Geometry check sheet. Reference: the model listing, model coordinates, mm. A direction names the side the tool comes from. Give positions to 0.01 mm unless a question says otherwise; leave off trailing zeros. Loops run counter-clockwise (first coordinate to the right, second up) from the corner with the lowest first, then second, coordinate; pieces in that order, holes last. Notation, with made-up numbers: (42.5, 51) -> (58.5, 51) arc R23 ccw to (58.5, 61) -> close; hole circle Ø1 at (36.5, 32.25). An arc over 180 degrees is marked (long way). Answer as a JSON object with one key per item and string values.
from build123d import *

# Parameters (mm, degrees)
BOSS_EXTRUDE1_DEPTH = 15
SKETCH2_R           = 10
BOSS_EXTRUDE2_DEPTH = 134
SKETCH4_R           = 7.25
CUT_EXTRUDE1_DEPTH  = 57
CUT_EXTRUDE2_DEPTH  = 93
SKETCH7_R           = 6.5
CUT_EXTRUDE3_DEPTH  = 6.6
SKETCH8_R           = 3.2
CUT_EXTRUDE4_DEPTH  = 9.4
FILLET1_R           = 0.25
CHAMFER1_SIZE       = 1
FILLET2_R           = 0.5
FILLET3_R           = 0.5
FILLET4_R           = 0.5
SKETCH9_R           = 3
CUT_EXTRUDE5_DEPTH  = 16
FILLET5_R           = 1


with BuildPart() as part:
    # Sketch1 → Boss-Extrude1 (new body)
    with BuildSketch(Plane(origin=(0, 0, 0), x_dir=(1, 0, 0), z_dir=(0, 1, 0))):
        with BuildLine():
            Line((17, -24.718414189), (17, 24.718414189))
            ThreePointArc((17, 24.718414189), (-30, 0), (17, -24.718414189))
        make_face()
    extrude(amount=BOSS_EXTRUDE1_DEPTH)

    # Sketch2 → Boss-Extrude2 (add)
    with BuildSketch(Plane(origin=(0, 15, 0), x_dir=(1, 0, 0), z_dir=(0, 1, 0))):
        Circle(SKETCH2_R)
    extrude(amount=BOSS_EXTRUDE2_DEPTH)

    # Sketch4 → Cut-Extrude1 (cut)
    with BuildSketch(Plane.XZ):
        Circle(SKETCH4_R)
    extrude(amount=-CUT_EXTRUDE1_DEPTH, mode=Mode.SUBTRACT)

    # Sketch5 → Cut-Extrude2 (cut, through all)
    with BuildSketch(Plane.XZ.offset(-57)):
        with BuildLine():
            Line((-4, 3), (4, 3))
            ThreePointArc((4, 3), (0, -5), (-4, 3))
        make_face()
    extrude(amount=-CUT_EXTRUDE2_DEPTH, mode=Mode.SUBTRACT)

    # Sketch7 → Cut-Extrude3 (cut)
    with BuildSketch(Plane(origin=(0, 15, 0), x_dir=(1, 0, 0), z_dir=(0, 1, 0))):
        with Locations((0, -20)):
            Circle(SKETCH7_R)
        with Locations((-20, 0)):
            Circle(SKETCH7_R)
        with Locations((0, 20)):
            Circle(SKETCH7_R)
    extrude(amount=-CUT_EXTRUDE3_DEPTH, mode=Mode.SUBTRACT)

    # Sketch8 → Cut-Extrude4 (cut, through all)
    with BuildSketch(Plane(origin=(0, 8.4, 0), x_dir=(1, 0, 0), z_dir=(0, 1, 0))):
        with Locations((0, -20)):
            Circle(SKETCH8_R)
        with Locations((-20, 0)):
            Circle(SKETCH8_R)
        with Locations((0, 20)):
            Circle(SKETCH8_R)
    extrude(amount=-CUT_EXTRUDE4_DEPTH, mode=Mode.SUBTRACT)

    # Fillet1
    fillet1_edges = [part.edges().sort_by_distance(p)[0] for p in [
        (4, 103, 3),
        (-4, 103, 3),
    ]]
    fillet(fillet1_edges, radius=FILLET1_R)

    # Chamfer1
    chamfer1_edges = [part.edges().sort_by_distance(p)[0] for p in [
        (17, 0, 0),
        (-30, 0, 0),
    ]]
    chamfer(chamfer1_edges, length=CHAMFER1_SIZE)

    # Fillet2
    fillet2_edges = [part.edges().sort_by_distance(p)[0] for p in [
        (-10, 149, 0),
    ]]
    fillet(fillet2_edges, radius=FILLET2_R)

    # Fillet3
    fillet3_edges = [part.edges().sort_by_distance(p)[0] for p in [
        (0, 149, 3),
        (0, 149, -5),
        (3.987691213, 149, 2.972130829),
        (-3.987691213, 149, 2.972130829),
    ]]
    fillet(fillet3_edges, radius=FILLET3_R)

    # Fillet4
    fillet4_edges = [part.edges().sort_by_distance(p)[0] for p in [
        (-10, 15, 0),
    ]]
    fillet(fillet4_edges, radius=FILLET4_R)

    # Sketch9 → Cut-Extrude5 (cut, through all)
    with BuildSketch(Plane(origin=(0, 15, 0), x_dir=(1, 0, 0), z_dir=(0, 1, 0))):
        with Locations((-14.142135624, -14.142135624)):
            Circle(SKETCH9_R)
    extrude(amount=-CUT_EXTRUDE5_DEPTH, mode=Mode.SUBTRACT)

    # Fillet5
    fillet5_edges = [part.edges().sort_by_distance(p)[0] for p in [
        (17, 8, -24.718414189),
        (17, 8, 24.718414189),
    ]]
    fillet(fillet5_edges, radius=FILLET5_R)


solid = part.part
1) Section check C-C on y = 13.5. Record the cut outline in (x, z).
Geometry check:
{"outline": "(16.55, -25.02) arc R1 ccw to (17, -24.19) -> (17, 24.19) arc R1 ccw to (16.55, 25.02) arc R30 ccw (long way) to start; hole circle Ø13 at (-20, 0); hole circle Ø6 at (-14.14, 14.14); hole circle Ø14.5 at (0, 0); hole circle Ø13 at (0, -20); hole circle Ø13 at (0, 20)"}
2) Draft check along X on faces 4 (the face through (17, 8, 0)), 5 (the face through (-7, 0, 6)), 6 (the face through (-26.494, 11.746, -0.286)). Enter one of: pulls with the +X half, pulls with the -X half, needs draft (parallel to the pull), parting line crosses it, or undercut.
Geometry check:
{"face 4": "pulls with the +X half", "face 5": "needs draft", "face 6": "undercut"}
3) Section check D-D on y = 49. Record the cut outline in (x, z).
Geometry check:
{"outline": "circle Ø20 at (0, 0); hole circle Ø14.5 at (0, 0)"}
4) Depth check by flat-ended pin: P1, Ø7.5, axis at x = 0, z = 20, coming from the -Y side; P2, Ø4, axis at x = -2.5, z = 18, coming from the +Y side; P3, Ø8, axis at x = -5.5, y = 84, coming from the +Z side; P4, Ø6, axis at x = -6, y = 58.5, coming from the +Z side. Enter the tip coordinate at first touch or a pass-through.
Geometry check:
{"P1": "stops at y = 0", "P2": "stops at y = 8.4", "P3": "stops at z = 9.89", "P4": "stops at z = 9.54"}
5) Material ranges on line 1 along Z through (x, y) = (0, 6); line 2 along Z through (x, y) = (0, 122); line 3 along Z through (x, y) = (0, 13.25), recorded low to high. Write a range as from..to.
Geometry check:
{"line 1": "z = -30..-23.2, -16.8..-7.25, 7.25..16.8, 23.2..30", "line 2": "z = -10..-5, 3..10", "line 3": "z = -30..-26.5, -13.5..-7.25, 7.25..13.5, 26.5..30"}
6) Section check B-B on x = 0. Count the separate pieces of the cut face and the enclosed holes in it, plus the area to 3 significant figures.
Geometry check:
{"separate pieces": "4", "enclosed holes": "0", "area": "1,740 mm2"}
7) Tool access check on faces 1 (the face through (3.35, 28.1, -6.43)), 2 (the face through (0, 102, 3)), 3 (the face through (-0.846, 11.746, -26.445)). Record the directions out of +Z, -Z, +X, -X, +Y, -Y that give a thin tool (end or side, any length) a straight path to the whole face; none if there is none.
Geometry check:
{"face 1": "-Y", "face 2": "+Y, -Y", "face 3": "+Y"}
8) Section check A-A on y = 84.5. Record the cut outline in (x, z).
Geometry check:
{"outline": "circle Ø20 at (0, 0); hole (-4.08, 2.89) arc R5 ccw (long way) to (4.08, 2.89) arc R0.25 ccw to (3.87, 3) -> (-3.87, 3) arc R0.25 ccw to start"}
